For this review, take the finished solid that the model builds, in its own axes (mm). Face numbers are marked on the shaded views. A direction names the side the tool comes from. Round coordinates to 2 decimals unless told otherwise and drop trailing zeros. Write each loop counter-clockwise with the first axis right and the second up, starting at its lowest first coordinate (ties: lowest second). Pieces come first, ordered by that corner, then holes. Notation, with made-up numbers: (-38, 38.25) -> (-7, 38.25) arc R21 cw to (-7, 50.25) -> close; hole circle Ø9 at (-31, -17). An arc over 180 degrees is marked (long way). Answer in a Markdown table with one row per item.
from build123d import *

# Parameters (mm, degrees)
BOSS_EXTRUDE1_DEPTH = 5
SKETCH4_R           = 0.8
CUT_EXTRUDE3_DEPTH  = 20.474342094
SKETCH5_W           = 4
SKETCH5_H           = 3
CUT_EXTRUDE4_DEPTH  = 13
FILLET4_R           = 1
CUT_EXTRUDE5_DEPTH  = 20.474342094
FILLET6_R           = 1
CUT_EXTRUDE6_START  = -8.5
CUT_EXTRUDE6_DEPTH  = 8.037702488
SKETCH11_W          = 3
SKETCH11_H          = 5
CUT_EXTRUDE8_DEPTH  = 4
SKETCH12_R          = 0.6
CUT_EXTRUDE9_DEPTH  = 5
CUT_EXTRUDE10_REACH = 21.474
SKETCH9_R           = 0.25


# Read off the part's stored shape, not the designer's step: Cut-Extrude6
with BuildPart() as part:
    # Sketch1 → Boss-Extrude1 (new body)
    with BuildSketch(Plane.XY):
        Polygon((0, 0), (12, 0), (12, -14.5), (6.5, -14.5), (6.5, -5), (0, -5), align=None)
    extrude(amount=BOSS_EXTRUDE1_DEPTH)

    # Sketch4 → Cut-Extrude3 (cut, through all)
    with BuildSketch(Plane.XY.offset(5)):
        with Locations((1.75, -2.5)):
            Circle(SKETCH4_R)
    extrude(amount=-CUT_EXTRUDE3_DEPTH, mode=Mode.SUBTRACT)

    # Sketch5 → Cut-Extrude4 (cut)
    with BuildSketch(Plane(origin=(0, 0, 0), x_dir=(1, 0, 0), z_dir=(0, 1, 0))):
        with Locations((2, -2.5)):
            Rectangle(SKETCH5_W, SKETCH5_H)
    extrude(amount=-CUT_EXTRUDE4_DEPTH, mode=Mode.SUBTRACT)

    # Fillet4
    fillet4_edges = [part.edges().sort_by_distance(p)[0] for p in [
        (0, 0, 4.5),
        (0, -5, 4.5),
        (0, 0, 0.5),
        (0, -5, 0.5),
    ]]
    fillet(fillet4_edges, radius=FILLET4_R)

    # Sketch6 → Cut-Extrude5 (cut, through all)
    with BuildSketch(Plane.XY.offset(5)):
        Polygon((12, -13.588182425), (11, -12.588182425), (12, -11.588182425), align=None)
    extrude(amount=-CUT_EXTRUDE5_DEPTH, mode=Mode.SUBTRACT)

    # Fillet6
    fillet6_edges = [part.edges().sort_by_distance(p)[0] for p in [
        (11, -12.588182425, 2.5),
        (12, -13.588182425, 2.5),
        (12, -11.588182425, 2.5),
        (6.5, -5, 2.5),
        (6.5, -14.5, 2.5),
        (12, 0, 2.5),
    ]]
    fillet(fillet6_edges, radius=FILLET6_R - 0.0001)  # a hair under: the kernel refuses the full size

    # Cut-Extrude6 outline → Cut-Extrude6 (cut)
    with BuildSketch(Plane.XZ.offset(14.5).offset(CUT_EXTRUDE6_START)):
        with BuildLine():
            Line((6.499992217, 5.000061772), (6.49999198, -6.3653e-05))
            ThreePointArc((6.49999198, -6.3653e-05), (6.656865167, 2.499999052), (6.499992217, 5.000061772))
        make_face()
    extrude(amount=CUT_EXTRUDE6_DEPTH, mode=Mode.SUBTRACT)

    # Sketch11 → Cut-Extrude8 (cut, along a direction that is not the sketch's normal)
    with BuildSketch(Plane.ZY.offset(-4)):
        with Locations((2.5, -2.5)):
            Rectangle(SKETCH11_W, SKETCH11_H)
    extrude(amount=-CUT_EXTRUDE8_DEPTH, dir=(-0.8191736087025463, 0.5735456379445732, 0), mode=Mode.SUBTRACT)

    # Sketch12 → Cut-Extrude9 (cut, along a direction that is not the sketch's normal)
    with BuildSketch(Plane.ZY.offset(-6.5)):
        with Locations((3.671694189, -8.375443102)):
            Circle(SKETCH12_R)
        with Locations((3.671694189, -10.194652501)):
            Circle(SKETCH12_R)
        with Locations((3.671694189, -12.168032187)):
            Circle(SKETCH12_R)
    extrude(amount=-CUT_EXTRUDE9_DEPTH, dir=(-0.8191736087025463, 0.5735456379445732, 0), mode=Mode.SUBTRACT)

    # Cut-Extrude10: up to this plane
    cut_extrude10_end = Plane(origin=(7.276694435, -7.294182552, 1), z_dir=(-0.5735456379445732, -0.8191736087025463, 0))
    # Sketch9 → Cut-Extrude10 (cut, up to the surface)
    with BuildSketch(Plane.XZ.offset(14.5), mode=Mode.PRIVATE) as cut_extrude10_sk1:
        with Locations((6.656865167, 2.5)):
            Circle(SKETCH9_R)
    cut_extrude10_tool1 = split(extrude(cut_extrude10_sk1.sketch, amount=-CUT_EXTRUDE10_REACH, mode=Mode.PRIVATE), bisect_by=cut_extrude10_end, keep=Keep.BOTH, mode=Mode.PRIVATE)
    add(cut_extrude10_tool1.solids().sort_by_distance((6.656865, -14.5, 2.5))[0], mode=Mode.SUBTRACT)


solid = part.part
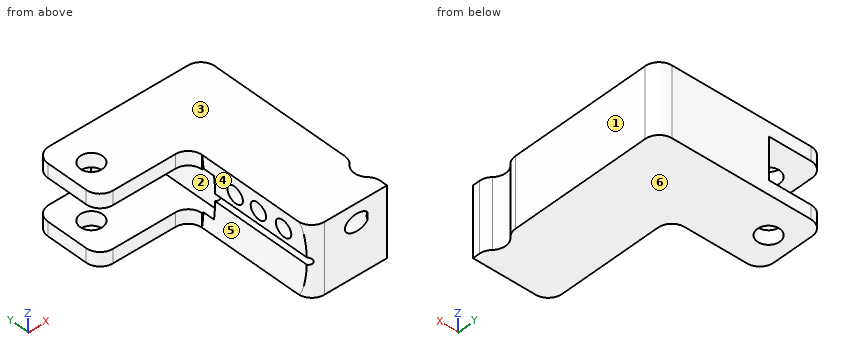
1) Mouldability with a two-part tool opening along Z and no side actions: class the marked faces 1, 2, 3 and 4 as pulls with the +Z half, pulls with the -Z half, needs draft (parallel to the pull), parting line crosses it, or undercut.
Solved:
| item | result |
|---|---|
| face 1 | needs draft |
| face 2 | undercut |
| face 3 | pulls with the +Z half |
| face 4 | undercut |
2) Consider section A-A on y = -2.5. State the section outline as (x, z) points.
Solved:
| item | result |
|---|---|
| outline | (0, 0) -> (0.95, 0) -> (0.95, 1) -> (0, 1) -> close; (0, 4) -> (0.95, 4) -> (0.95, 5) -> (0, 5) -> close; (2.55, 0) -> (12, 0) -> (12, 5) -> (2.55, 5) -> (2.55, 4) -> (7.28, 4) -> (7.28, 1) -> (2.55, 1) -> close |
3) Consider section B-B on x = 1.75. State the section outline as (y, z) points.
Solved:
| item | result |
|---|---|
| outline | (-5, 0) -> (-3.3, 0) -> (-3.3, 1) -> (-5, 1) -> close; (-5, 4) -> (-3.3, 4) -> (-3.3, 5) -> (-5, 5) -> close; (-1.7, 0) -> (0, 0) -> (0, 1) -> (-1.7, 1) -> close; (-1.7, 4) -> (0, 4) -> (0, 5) -> (-1.7, 5) -> close |
4) Clearance check with flat-ended pins moving along their axes: pin 1 Ø1.3 at (y, z) = (-11, 4) entering from -X; pin 2 Ø0.8 at (x, z) = (3, 0.5) entering from -Y; pin 3 Ø1 at (x, y) = (1.75, -2.5) entering from -Z. State where each tip first meets the part, or that it passes through.
Solved:
| item | result |
|---|---|
| pin 1 | x = 6.54 |
| pin 2 | y = -5 |
| pin 3 | through |
5) For the marked faces 5 and 6, list the 3-axis set-ups (+Z, -Z, +X, -X, +Y, -Y) from which the entire face can be reached by the end or side of a thin tool; tool diameter is ignored.
Solved:
| item | result |
|---|---|
| face 5 | -X, -Y |
| face 6 | -Z, +X, -X, +Y, -Y |
6) For line 1 (Y direction, x = 1.75, z = 0.55); line 2 (Z direction, x = 5.75, y = -5); line 3 (Y direction, x = 4, z = 4.1), list the stretches that pass through material, from the lowest coordinate up. Write a range as [from, to].
Solved:
| item | result |
|---|---|
| line 1 | [-5, -3.3], [-1.7, 0] |
| line 2 | [0, 1], [4, 5] |
| line 3 | [-5, 0] |
